Geometry: final body of the model. Coordinates: model frame, mm. A direction names the side the tool comes from. Coordinates: 2 decimals unless noted, no trailing zeros. Order: outer loops, then holes, each group sorted by start corner. A loop starts at its lowest first (then second) coordinate and runs counter-clockwise, first axis right, second up. Notation, with made-up numbers: (47.5, -10) - (94.5, -10) arc R26 ccw to (94.5, 22) - close; hole circle Ø1 at (74.5, 70.25). An arc over 180 degrees is marked (long way). Use one line per item in the form item = value. Start each with the question number.
```python
from build123d import *

# Parameters (mm, degrees)
F0_W     = 127
F0_H     = 69.85
F1_DEPTH = 6.35
F2_W     = 114.3
F2_H     = 63.5
F3_DEPTH = 6.35
F4_R     = 2.54


with BuildPart() as f1:
    # F0 (on Top) → F1 (new body)
    with BuildSketch(Plane.XY):
        Rectangle(F0_W, F0_H)
    extrude(amount=F1_DEPTH)

    # F2 (on face) → F3 (join, symmetric)
    with BuildSketch(Plane.XY.offset(6.35)):
        Rectangle(F2_W, F2_H)
    extrude(amount=F3_DEPTH, both=True)

    # F4
    f4_edges = [f1.edges().sort_by_distance(p)[0] for p in [
        (0, -34.925, 0),
        (-63.5, 0, 0),
        (-63.5, 0, 6.35),
        (-63.5, -34.925, 3.175),
        (0, -34.925, 6.35),
        (63.5, 0, 0),
        (63.5, 0, 6.35),
        (63.5, 34.925, 3.175),
        (0, 34.925, 6.35),
        (63.5, -34.925, 3.175),
        (0, 34.925, 0),
        (-63.5, 34.925, 3.175),
    ]]
    fillet(f4_edges, radius=F4_R)


solid = f1.part
```
(1) Material intervals for L1, parallel to X at y = -22.5, z = 4; L2, parallel to Z at x = 6.5, y = -32; L3, parallel to Y at x = -50, z = 12, sorted ascending. Write a range as from..to.
(2) Cut plane A-A on y = 11. Return the cut outline in (x, z).
(3) Cut plane B-B on x = -38. Return the cut outline in (y, z) (3 decimals).
(4) Set-up query: faces 1 (the flat face through (57.15, 0, 10)), 2 (the flat face through (-1, 31.75, 10)), 3 (the flat face through (-1, -31.75, 10)), 4 (the flat face through (-57.15, 0, 10)). Return all of +Z, -Z, +X, -X, +Y, -Y with unobstructed straight access to the full face (end or side cutting, diameter ignored); none if empty.
(5) Contact query for flat-ended pins moving along their axis: pin 1 Ø1 at (y, z) = (4, 1.5) entering from -X; pin 2 Ø1.9 at (y, z) = (3.5, 8.5) entering from -X; pin 3 Ø1.9 at (x, z) = (28.5, 9.5) entering from -Y. Output: stop coordinate, or through.
(6) Cut plane C-C on z = 9.5. Return the cut outline in (x, y), plus the area to 3 significant figures.
Check sheet entries:
q1.L1 = -63.49..63.49
q1.L2 = 0..6.35
q1.L3 = -31.75..31.75
q2.outline = (-63.5, 2.54) arc R2.54 ccw to (-60.96, 0) - (60.96, 0) arc R2.54 ccw to (63.5, 2.54) - (63.5, 3.81) arc R2.54 ccw to (60.96, 6.35) - (57.15, 6.35) - (57.15, 12.7) - (-57.15, 12.7) - (-57.15, 6.35) - (-60.96, 6.35) arc R2.54 ccw to (-63.5, 3.81) - close
q3.outline = (-34.925, 2.54) arc R2.54 ccw to (-32.385, 0) - (32.385, 0) arc R2.54 ccw to (34.925, 2.54) - (34.925, 3.81) arc R2.54 ccw to (32.385, 6.35) - (31.75, 6.35) - (31.75, 12.7) - (-31.75, 12.7) - (-31.75, 6.35) - (-32.385, 6.35) arc R2.54 ccw to (-34.925, 3.81) - close
q4.face_1 = +Z, +X, +Y, -Y
q4.face_2 = +Z, +X, -X, +Y
q4.face_3 = +Z, +X, -X, -Y
q4.face_4 = +Z, -X, +Y, -Y
q5.pin_1 = -63.44
q5.pin_2 = -57.15
q5.pin_3 = -31.75
q6.outline = (-57.15, -31.75) - (57.15, -31.75) - (57.15, 31.75) - (-57.15, 31.75) - close
q6.area = 7,260 mm^2
